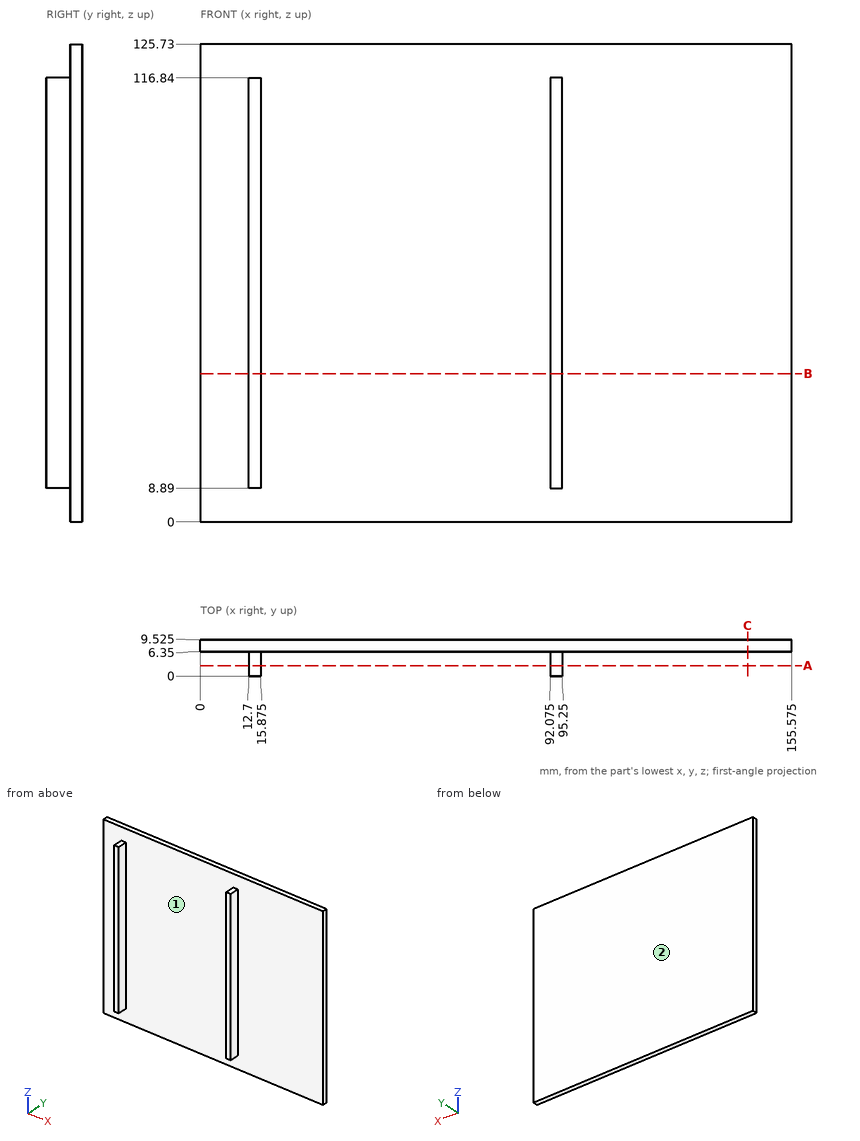
Verification items for this drawing (mm, ordinates from the low corner). Round coordinates to 2 decimals unless told otherwise and drop trailing zeros. Order: outer loops, then holes, each group sorted by start corner. A loop starts at its lowest first (then second) coordinate and runs counter-clockwise, first axis right, second up. Notation, with made-up numbers: (22, -21) -> (72, -21) arc R18 cw to (72, 1) -> close; hole circle Ø9 at (31, -6.75). An arc over 180 degrees is marked (long way). Use one line per item in the form item = value.
1. Scan lines: line 1 along X through (y, z) = (1.25, 81.5) (3 decimals); line 2 along Y through (x, z) = (26, 55) (3 decimals); line 3 along Z through (x, y) = (15, 1.75). Record each from-to range of solid material in increasing order. Write a range as from..to.
Working result:
line_1 = 12.7..15.875, 92.075..95.25
line_2 = 6.35..9.525
line_3 = 8.89..116.84
2. Cross-section at C-C, the plane x = 144. Enter the section's corners in (y, z) (3 decimals).
Working result:
outline = (6.35, 0) -> (9.525, 0) -> (9.525, 125.73) -> (6.35, 125.73) -> close
3. Go/stop test with flat-tipped pins: pin 1 (5 mm diameter, centred on x = 63, y = 2, fed in from +Z); pin 2 (3 mm diameter, centred on y = 3.5, z = 42.5, fed in from -X); pin 3 (1.9 mm diameter, centred on y = 4.5, z = 88.5, fed in from +X); pin 4 (1 mm diameter, centred on x = 14.5, y = 4.5, fed in from -Z). Record where each tip stops, or that it passes through.
Working result:
pin_1 = through
pin_2 = 12.7
pin_3 = 95.25
pin_4 = 8.89
4. Mould release check, pull along X, two halves, no side actions. Record for the marked faces 1 and 2: pulls with the +X half, pulls with the -X half, needs draft (parallel to the pull), parting line crosses it, or undercut.
Working result:
face_1 = undercut
face_2 = needs draft
5. Cross-section at B-B, the plane z = 39. Enter the section's corners in (x, y) (3 decimals).
Working result:
outline = (0, 6.35) -> (12.7, 6.35) -> (12.7, 0) -> (15.875, 0) -> (15.875, 6.35) -> (92.075, 6.35) -> (92.075, 0) -> (95.25, 0) -> (95.25, 6.35) -> (155.575, 6.35) -> (155.575, 9.525) -> (0, 9.525) -> close
6. Cross-section at A-A, the plane y = 2.75. Enter the section's corners in (x, z) (3 decimals), plus the area to 3 significant figures.
Working result:
outline = (12.7, 8.89) -> (15.875, 8.89) -> (15.875, 116.84) -> (12.7, 116.84) -> close; (92.075, 8.89) -> (95.25, 8.89) -> (95.25, 116.84) -> (92.075, 116.84) -> close
area = 685 mm^2
